For this review, take the finished solid that the model builds, in its own axes (mm). A direction names the side the tool comes from. Coordinates: 2 decimals unless noted, no trailing zeros. Loops run counter-clockwise (first coordinate to the right, second up) from the corner with the lowest first, then second, coordinate; pieces in that order, holes last. Notation, with made-up numbers: (24, -24) -> (48, -24) arc R14 ccw to (48, -4) -> close; hole circle Ø1 at (-9.5, -40). An arc over 180 degrees is marked (long way). Answer in a Markdown table with one row per item.
from build123d import *

# Parameters (mm, degrees)
SKETCH1_R           = 48.25
BOSS_EXTRUDE1_DEPTH = 5
SKETCH2_W           = 17.162038191
SKETCH2_H           = 56.822210482
SKETCH2_W_2         = 16.152506533
SKETCH2_H_2         = 65.186901365
CUT_EXTRUDE1_DEPTH  = 8
SKETCH3_R           = 30
CUT_EXTRUDE2_DEPTH  = 8
SKETCH4_R           = 1.75
CUT_EXTRUDE3_DEPTH  = 10
SKETCH9_R           = 3
CUT_EXTRUDE4_DEPTH  = 3.5
SKETCH12_R          = 48.25
BOSS_EXTRUDE4_DEPTH = 5
SKETCH13_W          = 17.162038191
SKETCH13_H          = 240.265998925
SKETCH13_W_2        = 16.152506533
SKETCH13_H_2        = 226.18217938
CUT_EXTRUDE5_DEPTH  = 5
SKETCH14_R          = 30
CUT_EXTRUDE6_DEPTH  = 5
CUT_EXTRUDE7_DEPTH  = 5
CUT_EXTRUDE8_DEPTH  = 5
SKETCH19_R          = 1.75
CUT_EXTRUDE9_DEPTH  = 5
SKETCH20_R          = 3
CUT_EXTRUDE10_DEPTH = 3.5
BOSS_EXTRUDE5_DEPTH = 5
SKETCH21_R          = 30
CUT_EXTRUDE11_DEPTH = 5
SKETCH22_R          = 3
CUT_EXTRUDE12_DEPTH = 3.5


with BuildPart() as part:
    # Sketch1 → Boss-Extrude1 (new body)
    with BuildSketch(Plane.XY):
        Circle(SKETCH1_R)
    extrude(amount=-BOSS_EXTRUDE1_DEPTH)

    # Sketch2 → Cut-Extrude1 (cut)
    with BuildSketch(Plane.XY):
        with Locations((-54.831019095, 0)):
            Rectangle(SKETCH2_W, SKETCH2_H)
        with Locations((54.326253267, -4.182345442)):
            Rectangle(SKETCH2_W_2, SKETCH2_H_2)
    extrude(amount=-CUT_EXTRUDE1_DEPTH, mode=Mode.SUBTRACT)

    # Sketch3 → Cut-Extrude2 (cut)
    with BuildSketch(Plane.XY):
        Circle(SKETCH3_R)
    extrude(amount=-CUT_EXTRUDE2_DEPTH, mode=Mode.SUBTRACT)

    # Sketch4 → Cut-Extrude3 (cut)
    with BuildSketch(Plane.XY):
        with Locations((-42.5, 0)):
            Circle(SKETCH4_R)
        with Locations((0, -44.5)):
            Circle(SKETCH4_R)
        with Locations((0, 44.5)):
            Circle(SKETCH4_R)
        with Locations((42.5, 0)):
            Circle(SKETCH4_R)
        with Locations((-31.466251763, -31.466251763)):
            Circle(SKETCH4_R)
        with Locations((31.466251763, -31.466251763)):
            Circle(SKETCH4_R)
        with Locations((31.466251763, 31.466251763)):
            Circle(SKETCH4_R)
        with Locations((-31.466251763, 31.466251763)):
            Circle(SKETCH4_R)
    extrude(amount=-CUT_EXTRUDE3_DEPTH, mode=Mode.SUBTRACT)

    # Sketch9 → Cut-Extrude4 (cut)
    with BuildSketch(Plane.XY):
        with Locations((-42.5, 0)):
            Circle(SKETCH9_R)
        with Locations((42.5, 0)):
            Circle(SKETCH9_R)
        with Locations((31.466251763, 31.466251763)):
            Circle(SKETCH9_R)
        with Locations((-31.466251763, 31.466251763)):
            Circle(SKETCH9_R)
        with Locations((-31.466251763, -31.466251763)):
            Circle(SKETCH9_R)
        with Locations((31.466251763, -31.466251763)):
            Circle(SKETCH9_R)
        with Locations((0, -44.5)):
            Circle(SKETCH9_R)
        with Locations((0, 44.5)):
            Circle(SKETCH9_R)
    extrude(amount=-CUT_EXTRUDE4_DEPTH, mode=Mode.SUBTRACT)

    # Sketch17 → Cut-Extrude7 (cut)
    with BuildSketch(Plane.XY):
        Polygon((0, 0), (-69.304284442, 39.961433382), (-69.278270797, -65.322297693), (63.970930278, -62.407226987), (69.259758702, 40.038554227), align=None)
    extrude(amount=-CUT_EXTRUDE7_DEPTH, mode=Mode.SUBTRACT)



with BuildPart() as body_2:
    # Sketch12 → Boss-Extrude4 (new body)
    with BuildSketch(Plane.XY):
        with Locations((0, 304.453033425)):
            Circle(SKETCH12_R)
    extrude(amount=-BOSS_EXTRUDE4_DEPTH)

    # Sketch13 → Cut-Extrude5 (cut)
    with BuildSketch(Plane.XY):
        with Locations((-54.831019095, 316.834631882)):
            Rectangle(SKETCH13_W, SKETCH13_H)
        with Locations((54.326253267, 300.281083797)):
            Rectangle(SKETCH13_W_2, SKETCH13_H_2)
    extrude(amount=-CUT_EXTRUDE5_DEPTH, mode=Mode.SUBTRACT)

    # Sketch14 → Cut-Extrude6 (cut)
    with BuildSketch(Plane.XY):
        with Locations((0, 304.453033425)):
            Circle(SKETCH14_R)
    extrude(amount=-CUT_EXTRUDE6_DEPTH, mode=Mode.SUBTRACT)

    # Sketch18 → Cut-Extrude8 (cut)
    with BuildSketch(Plane.XY):
        Polygon((0, 304.453033425), (-69.251773631, 264.400669588), (-69.066382196, 357.511219566), (54.70167511, 362.333351669), (69.31225138, 264.505420122), align=None)
    extrude(amount=-CUT_EXTRUDE8_DEPTH, mode=Mode.SUBTRACT)

    # Sketch19 → Cut-Extrude9 (cut)
    with BuildSketch(Plane.XY):
        with Locations((0, 259.953033425)):
            Circle(SKETCH19_R)
        with Locations((-31.466251763, 272.986781662)):
            Circle(SKETCH19_R)
        with Locations((31.466251763, 272.986781662)):
            Circle(SKETCH19_R)
    extrude(amount=-CUT_EXTRUDE9_DEPTH, mode=Mode.SUBTRACT)

    # Sketch20 → Cut-Extrude10 (cut)
    with BuildSketch(Plane.XY):
        with Locations((-31.466251763, 272.986781662)):
            Circle(SKETCH20_R)
        with Locations((0, 259.953033425)):
            Circle(SKETCH20_R)
        with Locations((31.466251763, 272.986781662)):
            Circle(SKETCH20_R)
    extrude(amount=-CUT_EXTRUDE10_DEPTH, mode=Mode.SUBTRACT)


with BuildPart() as part_1:
    add(part.part)

    add(body_2.part)  # Boss-Extrude5 merges body 2
    # Sketch10 → Boss-Extrude5 (add)
    # profile 1 of 4: a face of its own
    with BuildSketch(Plane.XY):
        with BuildLine():
            Line((-17.5, 243.53997423), (-17.5, 259.48846404))
            ThreePointArc((-17.5, 259.48846404), (-23.743486454, 262.449350837), (-29.5, 266.271722552))
            Line((-29.5, 266.271722552), (-29.5, 38.181310873))
            ThreePointArc((-29.5, 38.181310873), (-16.697131744, 45.268844601), (-2.358379682, 48.192328697))
            Line((-2.358379682, 48.192328697), (17.5, 59.53997423))
            Line((17.5, 59.53997423), (17.5, 44.964569385))
            ThreePointArc((17.5, 44.964569385), (23.743486454, 42.003682588), (29.5, 38.181310873))
            Line((29.5, 38.181310873), (29.5, 266.271722552))
            ThreePointArc((29.5, 266.271722552), (17.999468175, 259.686062951), (5.141024697, 256.477702628))
            Line((5.141024697, 256.477702628), (-17.5, 243.53997423))
        make_face()
        Polygon((17.5, 251.53997423), (17.5, 211.53997423), (-17.5, 231.53997423), align=None, mode=Mode.SUBTRACT)
        Polygon((17.5, 187.53997423), (17.5, 147.53997423), (-17.5, 167.53997423), align=None, mode=Mode.SUBTRACT)
        Polygon((-17.5, 179.53997423), (-17.5, 219.53997423), (17.5, 199.53997423), align=None, mode=Mode.SUBTRACT)
        Polygon((17.5, 135.53997423), (-17.5, 115.53997423), (-17.5, 155.53997423), align=None, mode=Mode.SUBTRACT)
        Polygon((17.5, 123.53997423), (17.5, 83.53997423), (-17.5, 103.53997423), align=None, mode=Mode.SUBTRACT)
        Polygon((17.5, 71.53997423), (-17.5, 51.53997423), (-17.5, 91.53997423), align=None, mode=Mode.SUBTRACT)
    # profile 2 of 4: a face of its own
    with BuildSketch(Plane.XY):
        with BuildLine():
            ThreePointArc((29.101447707, 274.83277781), (28.479675874, 272.7032954), (29.490995443, 270.728826288))
            ThreePointArc((29.490995443, 270.728826288), (29.367996239, 272.787614912), (29.101447707, 274.83277781))
        make_face()
    # profile 3 of 4: a face of its own
    with BuildSketch(Plane.XY):
        with BuildLine():
            ThreePointArc((-29.101447707, 274.83277781), (-29.367996239, 272.787614912), (-29.490995443, 270.728826288))
            ThreePointArc((-29.490995443, 270.728826288), (-28.479675874, 272.7032954), (-29.101447707, 274.83277781))
        make_face()
    # profile 4 of 4: a face of its own
    with BuildSketch(Plane.XY):
        with BuildLine():
            ThreePointArc((-24.25254041, 286.794769533), (0, 274.453033425), (24.25254041, 286.794769533))
            ThreePointArc((24.25254041, 286.794769533), (0, 299.5), (-24.25254041, 286.794769533))
        make_face()
    extrude(amount=-BOSS_EXTRUDE5_DEPTH)

    # Sketch21 → Cut-Extrude11 (cut)
    with BuildSketch(Plane.XY):
        with Locations((0, 304.453033425)):
            Circle(SKETCH21_R)
    extrude(amount=-CUT_EXTRUDE11_DEPTH, mode=Mode.SUBTRACT)

    # Sketch22 → Cut-Extrude12 (cut)
    with BuildSketch(Plane.XY):
        with Locations((31.466251763, 272.986781662)):
            Circle(SKETCH22_R)
        with Locations((-31.466251763, 272.986781662)):
            Circle(SKETCH22_R)
    extrude(amount=-CUT_EXTRUDE12_DEPTH, mode=Mode.SUBTRACT)


solid = part_1.part
Item 1: Insertion check: pin 1 (1.5 mm diameter, centred on y = 126.5, z = -3, fed in from -X); pin 2 (1.5 mm diameter, centred on y = 134, z = -3, fed in from +X); pin 3 (3 mm diameter, centred on x = 0, y = 259.95, fed in from -Z); pin 4 (5 mm diameter, centred on x = 31.47, y = 272.99, fed in from -Z). Each pin has a flat end and moves straight along its axis. Give the tip position at first contact, or say it passes through.
Worked answers:
| item | result |
|---|---|
| pin 1 | x = -29.5 |
| pin 2 | x = 29.5 |
| pin 3 | through |
| pin 4 | z = -5 |
Item 2: Take a section at C-C, the plane y = 150. State the section outline as (x, z) points.
Worked answers:
| item | result |
|---|---|
| outline | (-29.5, -5) -> (-17.5, -5) -> (-17.5, 0) -> (-29.5, 0) -> close; (-7.81, -5) -> (13.19, -5) -> (13.19, 0) -> (-7.81, 0) -> close; (17.5, -5) -> (29.5, -5) -> (29.5, 0) -> (17.5, 0) -> close |
Item 3: Take a section at B-B, the plane y = 110. State the section outline as (x, z) points, and give its area (3 significant figures).
Worked answers:
| item | result |
|---|---|
| outline | (-29.5, -5) -> (-6.19, -5) -> (-6.19, 0) -> (-29.5, 0) -> close; (17.5, -5) -> (29.5, -5) -> (29.5, 0) -> (17.5, 0) -> close |
| area | 177 mm² |
Item 4: For L1, parallel to X at y = 123, z = -2; L2, parallel to X at y = 218, z = -4; L3, parallel to Y at x = 33, z = -0.75, list the stretches that pass through material, from the lowest coordinate up.
Worked answers:
| item | result |
|---|---|
| L1 | -29.5 to -17.5, -4.44 to 16.56, 17.5 to 29.5 |
| L2 | -29.5 to -17.5, -14.81 to 6.19, 17.5 to 29.5 |
| L3 | 19.08 to 28.89, 34.04 to 35.2, 269.25 to 270.41, 275.57 to 285.43 |
Item 5: Take a section at A-A, the plane x = -9.5. Count the separate pieces of the cut face and the enclosed holes in it, and give its area (3 significant figures).
Worked answers:
| item | result |
|---|---|
| separate pieces | 8 |
| enclosed holes | 0 |
| area | 593 mm² |
Item 6: The part is to be moulded in two halves that separate along X. For faces 1 (the flat face through (-1, 154, -5)), 2 (the cylindrical face through (36.25, 272.61, -2.46)), 3 (the flat face through (-0.245, 81.68, -2.465)), say which applies: +X half, -X half, draft (parallel to the pull), parting line (faces both ways), or undercut.
Worked answers:
| item | result |
|---|---|
| face 1 | draft |
| face 2 | +X half |
| face 3 | undercut |
Item 7: For faces 4 (the flat face through (-30, 30, -3.5)), 5 (the flat face through (29.5, 151, -2)), 6 (the flat face through (-33.78, 19.48, -2.46)), 7 (the cylindrical face through (-0.417, 274.456, -2.465)), 8 (the flat face through (-0.245, 177.4, -2.465)), list the 3-axis set-ups (+Z, -Z, +X, -X, +Y, -Y) from which the entire face can be reached by the end or side of a thin tool; tool diameter is ignored.
Worked answers:
| item | result |
|---|---|
| face 4 | +Z |
| face 5 | +Z, -Z, +X |
| face 6 | +Z, -Z, -X, -Y |
| face 7 | +Z, -Z, +Y |
| face 8 | +Z, -Z |
